```python
from build123d import *

# Parameters (mm, degrees)
F0_W      = 4
F0_H      = 5
F0_R      = 3
F0_R_2    = 1.75
F1_DEPTH  = 5
F2_DEPTH  = 7
F3_START  = 2
F1_FACE_R = 1.75
F3_DEPTH  = 6.5
F4_SIZE   = 2.5
F5_START  = 5
F5_DEPTH  = 1.5
F6_R      = 5


with BuildPart() as f1:
    # F0 (on Top) → F1 (new body)
    with BuildSketch(Plane.XY):
        Polygon((21.9938950613, 39.5450913161), (-23.0061049387, 39.5450913161), (-23.0061049387, 19.5450913161), (-9.9312635139, 19.5450913161), (10.0687364861, 19.5450913161), (21.9938950613, 19.5450913161), align=None)
        Polygon((-12.5061049387, 32.0450913161), (-12.5061049387, 37.0450913161), (19.4938950613, 37.0450913161), (19.4938950613, 22.0450913161), (-12.5061049387, 22.0450913161), (-12.5061049387, 27.0450913161), (-16.5061049387, 27.0450913161), (-20.5061049387, 27.0450913161), (-20.5061049387, 32.0450913161), (-16.5061049387, 32.0450913161), align=None, mode=Mode.SUBTRACT)
        with Locations((-18.5061049387, 29.5450913161)):
            Rectangle(F0_W, F0_H)
        with Locations((-14.5061049387, 29.5450913161)):
            Rectangle(F0_W, F0_H)
        Polygon((19.4938950613, 37.0450913161), (-12.5061049387, 37.0450913161), (-12.5061049387, 32.0450913161), (-12.5061049387, 27.0450913161), (-12.5061049387, 22.0450913161), (19.4938950613, 22.0450913161), align=None)
        with Locations((10.4938950613, 30.0450913161)):
            Circle(F0_R, mode=Mode.SUBTRACT)
        with Locations((10.4938950613, 30.0450913161)):
            Circle(F0_R)
        with Locations((10.4938950613, 30.0450913161)):
            Circle(F0_R_2, mode=Mode.SUBTRACT)
    extrude(amount=F1_DEPTH)

    # F0 (on Top) → F2 (join)
    with BuildSketch(Plane.XY):
        Polygon((21.9938950613, 39.5450913161), (-23.0061049387, 39.5450913161), (-23.0061049387, 19.5450913161), (-9.9312635139, 19.5450913161), (10.0687364861, 19.5450913161), (21.9938950613, 19.5450913161), align=None)
        Polygon((-12.5061049387, 32.0450913161), (-12.5061049387, 37.0450913161), (19.4938950613, 37.0450913161), (19.4938950613, 22.0450913161), (-12.5061049387, 22.0450913161), (-12.5061049387, 27.0450913161), (-16.5061049387, 27.0450913161), (-20.5061049387, 27.0450913161), (-20.5061049387, 32.0450913161), (-16.5061049387, 32.0450913161), align=None, mode=Mode.SUBTRACT)
    extrude(amount=F2_DEPTH)

    # F0 (on Top) + F1_face (on face) → F3 (cut)
    with BuildSketch(Plane.XY.offset(F3_START)):
        with Locations((-18.5061049387, 29.5450913161)):
            Rectangle(F0_W, F0_H)
        with Locations((-14.5061049387, 29.5450913161)):
            Rectangle(F0_W, F0_H)
    with BuildSketch(Plane(origin=(1.7944753963, 29.5356658402, 5), x_dir=(1, 0, 0), z_dir=(0, 0, 1)).offset(F3_START)):
        Polygon((-22.300580335, -2.4905745241), (-14.300580335, -2.4905745241), (-14.300580335, -7.4905745241), (17.699419665, -7.4905745241), (17.699419665, 7.5094254759), (-14.300580335, 7.5094254759), (-14.300580335, 2.5094254759), (-22.300580335, 2.5094254759), align=None)
        with Locations((8.699419665, 0.5094254759)):
            Circle(F1_FACE_R, mode=Mode.SUBTRACT)
    extrude(amount=F3_DEPTH, mode=Mode.SUBTRACT)

    # F4
    f4_edges = [f1.edges().sort_by_distance(p)[0] for p in [
        (8.743895, 30.045091, 0),
    ]]
    chamfer(f4_edges, length=F4_SIZE)

    # F0 (on Top) → F5 (join)
    with BuildSketch(Plane.XY.offset(F5_START)):
        with Locations((10.4938950613, 30.0450913161)):
            Circle(F0_R)
        with Locations((10.4938950613, 30.0450913161)):
            Circle(F0_R_2, mode=Mode.SUBTRACT)
    extrude(amount=F5_DEPTH)

    # F6
    f6_edges = [f1.edges().sort_by_distance(p)[0] for p in [
        (-23.006105, 39.545091, 3.5),
    ]]
    fillet(f6_edges, radius=F6_R)


solid = f1.part
```
The listing builds one solid part. Answer for the finished solid, in the listing's coordinates (mm). A direction names the side the tool comes from. Coordinates: 2 decimals unless noted, no trailing zeros. Order: outer loops, then holes, each group sorted by start corner. A loop starts at its lowest first (then second) coordinate and runs counter-clockwise, first axis right, second up. Notation, with made-up numbers: M 81.5,15.25 L 115.5,15.25 A10 ccw 115.5,26.25 Z; hole C 16.25,51.5 d3. An arc over 180 degrees is marked long. Answer as a JSON object with one key per item and string values. Group by question number.
1. Determine the mould class of faces 1 (the flat face through (-7, 38, 7)), 2 (the flat face through (-16, 27.045, 4)), 3 (the flat face through (-23.006, 27, 3)) for opening direction X: released by +X, released by -X, zero draft, split by the parting line, or undercut.
2. Section B-B on x = 1.5 is taken. Write down the section's boundary in (y, z), then the cut area to 3 significant figures.
3. Straight lines are drawn through the part: line 1 (Y direction, x = -13, z = 4.25); line 2 (X direction, y = 30.75, z = 6.75); line 3 (X direction, y = 27.25, z = 2.5). For each, find the intervals that lie inside material, in ascending order.
4. A tool of negligible diameter and unlimited length cuts with its end or side. For faces 4 (the conical face through (12.22, 29.33, 2.38)), 5 (the flat face through (-17, 32.045, 4)), from which of +Z, -Z, +X, -X, +Y, -Y can it reach the whole face along a straight path? Write none if from no direction.
5. Flat-ended cylindrical pins translate along their axes: P1, Ø4.5, axis at x = 6, y = 27, coming from the +Z side; P2, Ø6.5, axis at x = 11.5, y = 30, coming from the +Z side; P3, Ø2, axis at x = 8, y = 31, coming from the -Z side. Find the tip coordinate at first contact, or state that the pin passes through.
6. Section A-A on y = 24 is taken. Write down the section's boundary in (x, z).
7. Section C-C on z = 3.25 is taken. Write down the section's boundary in (x, y), then the cut area to 3 significant figures.
8. Section D-D on z = 5.5 is taken. Write down the section's boundary in (x, y).
Values follow:
{
 "1": {"face 1": "zero draft", "face 2": "undercut", "face 3": "released by -X"},
 "2": {"outline": "M 19.55,0 L 39.55,0 L 39.55,7 L 37.05,7 L 37.05,5 L 22.05,5 L 22.05,7 L 19.55,7 Z", "area": "110 mm2"},
 "3": {"line 1": "19.55 to 27.05, 32.05 to 39.55", "line 2": "-23.01 to -20.51, 19.49 to 21.99", "line 3": "-23.01 to -20.51, -12.51 to 21.99"},
 "4": {"face 4": "-Z", "face 5": "+Z"},
 "5": {"P1": "z = 5", "P2": "z = 6.5", "P3": "z = 0.58"},
 "6": {"outline": "M -23.01,0 L 21.99,0 L 21.99,7 L 19.49,7 L 19.49,5 L -12.51,5 L -12.51,7 L -23.01,7 Z"},
 "7": {"outline": "M -23.01,19.55 L 21.99,19.55 L 21.99,39.55 L -18.01,39.55 A5 ccw -23.01,34.55 Z; hole M -20.51,27.05 L -12.51,27.05 L -12.51,32.05 L -20.51,32.05 Z; hole C 10.49,30.05 d3.5", "area": "845 mm2"},
 "8": {"outline": "M -23.01,19.55 L 21.99,19.55 L 21.99,39.55 L -18.01,39.55 A5 ccw -23.01,34.55 Z; C 10.49,30.05 d6; hole M -20.51,27.05 L -12.51,27.05 L -12.51,22.05 L 19.49,22.05 L 19.49,37.05 L -12.51,37.05 L -12.51,32.05 L -20.51,32.05 Z; hole C 10.49,30.05 d3.5"}
}
